Answer from the drawing. Dimensions are ordinates in mm from the lowest x, y and z of the part. A direction names the side the tool comes from. Round coordinates to 2 decimals unless told otherwise and drop trailing zeros. Loops run counter-clockwise (first coordinate to the right, second up) from the corner with the lowest first, then second, coordinate; pieces in that order, holes last. Notation, with made-up numbers: (81, 58) - (102, 58) arc R21 ccw to (102, 82) - close; hole circle Ø8 at (10.25, 81.25). An arc over 180 degrees is marked (long way). Answer as CSV lines item,"result". Start each with the question number.
Q1. Section B-B on x = 15.25 is taken. Write down the section's boundary in (y, z), then the cut area to 3 significant figures.
Q2. For the marked faces 5 and 6, determine the directions among +Z, -Z, +X, -X, +Y, -Y from which every point of the face is accessible in a straight line to the end or side of a thin tool.
Q3. Straight lines are drawn through the part: L1, parallel to Z at x = 8, y = 5; L2, parallel to Z at x = 8, y = 12.25; L3, parallel to Z at x = 7.25, y = 7.75 (1 decimal). For each, find the intervals that lie inside material, in ascending order. Write a range as [from, to].
Q4. Section A-A on y = 12.5 is taken. Write down the section's boundary in (x, z) (1 decimal).
Q5. Each of these flat-tipped pins is pushed along its axis until it touches: pin 1 Ø2.5 at (x, y) = (8, 13) entering from -Z; pin 2 Ø5 at (y, z) = (1.5, 17) entering from -X; pin 3 Ø8 at (x, z) = (8, 6) entering from -Y; pin 4 Ø2 at (y, z) = (4.5, 16) entering from -X. Where does it stop, or does it pass through?
Q6. Section C-C on z = 22 is taken. Write down the section's boundary in (x, y), then the cut area to 3 significant figures.
Q7. The mould has two halves that part along X. Classify the marked faces 1, 2, 3 and 4: +X half, -X half, draft (parallel to the pull), parting line (faces both ways), or undercut.
Q8. Section D-D on x = 3.5 is taken. Write down the section's boundary in (y, z) (1 decimal).
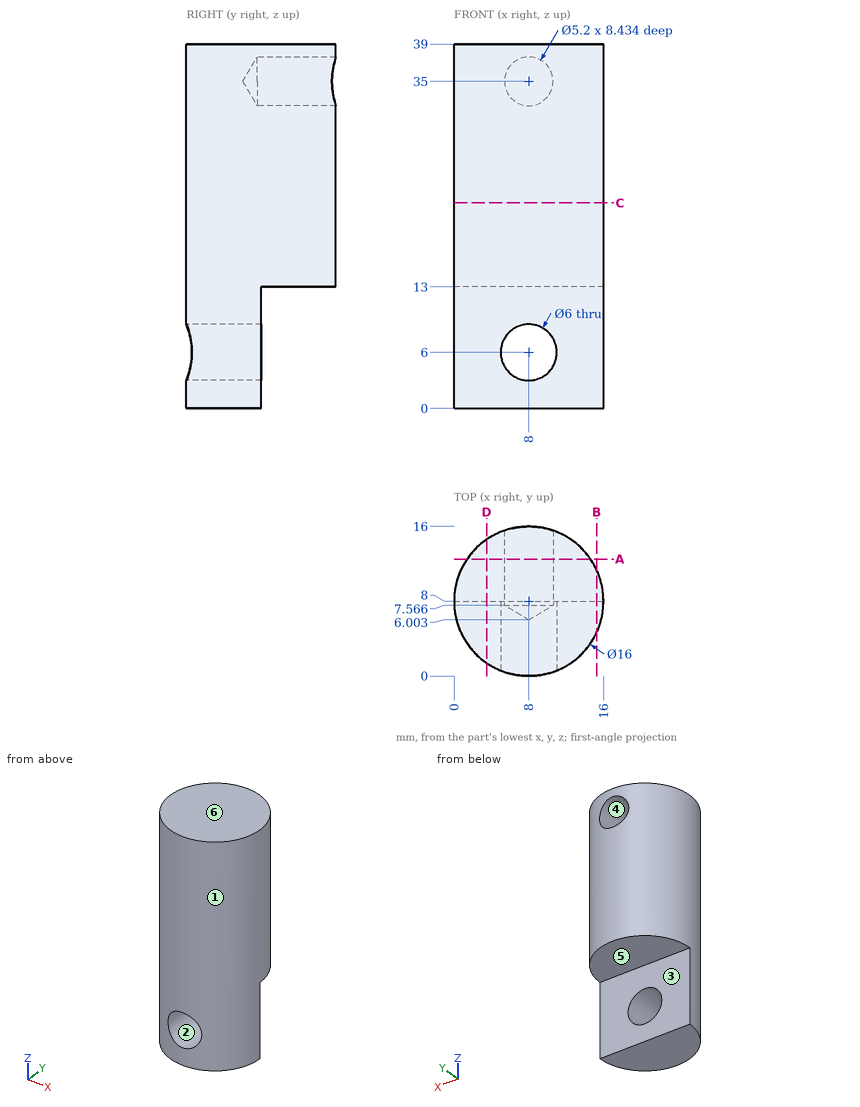
Findings:
1,outline,"(4.62, 0) - (8, 0) - (8, 13) - (11.38, 13) - (11.38, 39) - (4.62, 39) - close"
1,area,"220 mm^2"
2,face 5,"-Z, +X, -X, +Y"
2,face 6,"+Z, +X, -X, +Y, -Y"
3,L1,"z = [0, 3], [9, 39]"
3,L2,"z = [13, 32.4], [37.6, 39]"
3,L3,"z = [0, 3.1], [8.9, 32.5], [37.5, 39]"
4,outline,"(1.4, 13) - (14.6, 13) - (14.6, 39) - (1.4, 39) - close; hole circle Ø5.2 at (8, 35)"
5,pin 1,"stops at z = 13"
5,pin 2,"stops at x = 1.07"
5,pin 3,"stops at y = 0"
5,pin 4,"stops at x = 0.4"
6,outline,"circle Ø16 at (8, 8)"
6,area,"201 mm^2"
7,face 1,"parting line"
7,face 2,"undercut"
7,face 3,"draft"
7,face 4,"undercut"
8,outline,"(1.4, 0) - (8, 0) - (8, 13) - (14.6, 13) - (14.6, 39) - (1.4, 39) - close"
